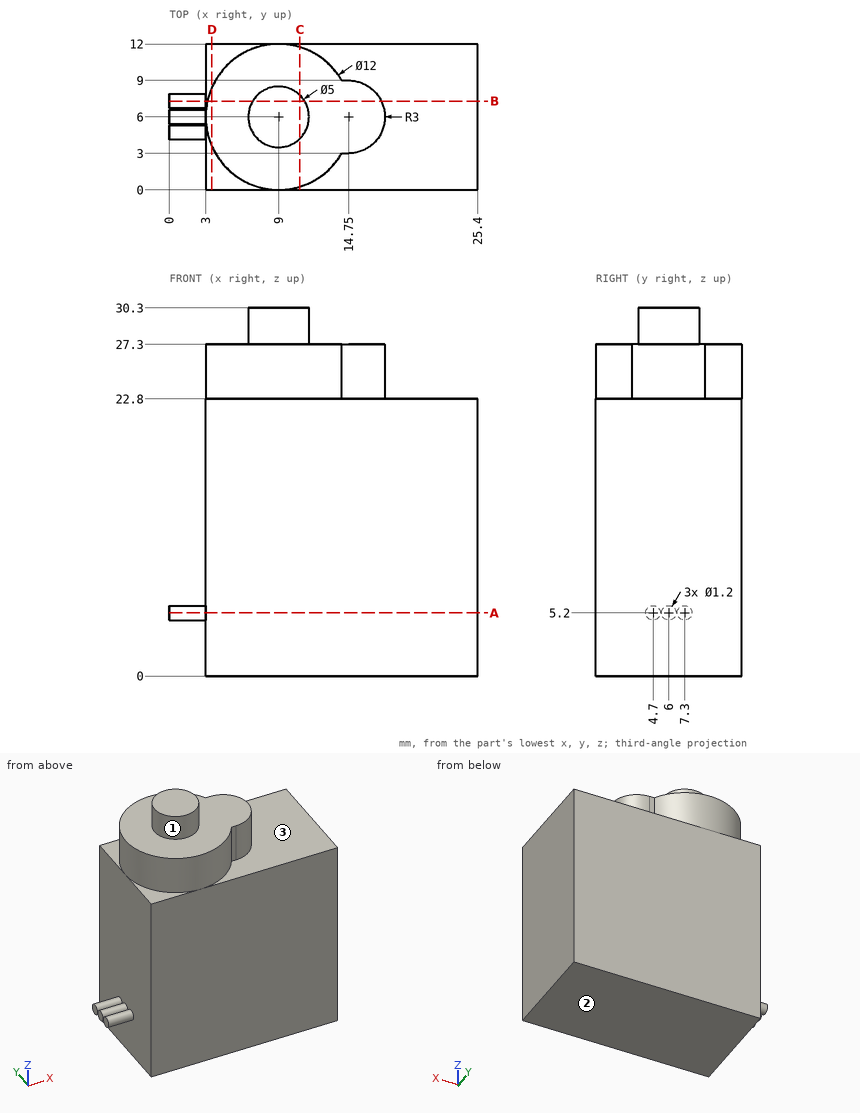
Answer from the drawing. Dimensions are ordinates in mm from the lowest x, y and z of the part. A direction names the side the tool comes from. Round coordinates to 2 decimals unless told otherwise and drop trailing zeros. Write each loop counter-clockwise with the first axis right and the second up, starting at its lowest first coordinate (ties: lowest second). Pieces come first, ordered by that corner, then holes. Notation, with made-up numbers: (82.5, -35) -> (123.5, -35) arc R17 cw to (123.5, -9) -> close; hole circle Ø9 at (-17, -33). An arc over 180 degrees is marked (long way). Write each question's results on one line, items separated by ' | '.
1) Which of the six approach directions +Z, -Z, +X, -X, +Y, -Y give full straight-line access (tool end or side, diameter ignored) to the marked faces 1, 2 and 3?
Findings:
face 1: +Z | face 2: -Z, +X, -X, +Y, -Y | face 3: +Z, +X
2) The part is cut by section D-D (x = 3.5). Write down the section's boundary in (y, z), and give its area (3 significant figures).
Findings:
outline: (0, 0) -> (12, 0) -> (12, 22.8) -> (8.4, 22.8) -> (8.4, 27.3) -> (3.6, 27.3) -> (3.6, 22.8) -> (0, 22.8) -> close | area: 295 mm²
3) The part is cut by section C-C (x = 10.75). Write down the section's boundary in (y, z).
Findings:
outline: (0, 0) -> (12, 0) -> (12, 22.8) -> (11.74, 22.8) -> (11.74, 27.3) -> (7.79, 27.3) -> (7.79, 30.3) -> (4.21, 30.3) -> (4.21, 27.3) -> (0.26, 27.3) -> (0.26, 22.8) -> (0, 22.8) -> close
4) The part is cut by section B-B (y = 7.3). Write down the section's boundary in (x, z), and give its area (3 significant figures).
Findings:
outline: (0, 4.6) -> (3, 4.6) -> (3, 0) -> (25.4, 0) -> (25.4, 22.8) -> (17.45, 22.8) -> (17.45, 27.3) -> (11.14, 27.3) -> (11.14, 30.3) -> (6.86, 30.3) -> (6.86, 27.3) -> (3.14, 27.3) -> (3.14, 22.8) -> (3, 22.8) -> (3, 5.8) -> (0, 5.8) -> close | area: 592 mm²
5) The part is cut by section A-A (z = 5.2). Write down the section's boundary in (x, y).
Findings:
outline: (0, 4.1) -> (3, 4.1) -> (3, 0) -> (25.4, 0) -> (25.4, 12) -> (3, 12) -> (3, 7.9) -> (0, 7.9) -> (0, 6.7) -> (3, 6.7) -> (3, 6.6) -> (0, 6.6) -> (0, 5.4) -> (3, 5.4) -> (3, 5.3) -> (0, 5.3) -> close
6) Consider line 1 along Z through (x, y) = (4.75, 6.5); line 2 along X through (y, z) = (8.25, 15.5); line 3 along Z through (x, y) = (19.25, 4). Determine where each line is inside the solid, lowest interval first. Write a range as [from, to].
Findings:
line 1: z = [0, 27.3] | line 2: x = [3, 25.4] | line 3: z = [0, 22.8]
7) Flat-ended cylindrical pins translate along their axes: pin 1 (6 mm diameter, centred on y = 3.5, z = 11, fed in from -X); pin 2 (3 mm diameter, centred on y = 1.5, z = 24.5, fed in from -X); pin 3 (6 mm diameter, centred on x = 12.5, y = 8, fed in from +Z); pin 4 (1.5 mm diameter, centred on x = 4, y = 8.5, fed in from +Z). Find the tip coordinate at first contact, or state that the pin passes through.
Findings:
pin 1: stops at x = 3 | pin 2: stops at x = 3.8 | pin 3: stops at z = 30.3 | pin 4: stops at z = 27.3
